Autodesk Inventor part; units mm, degrees
ref_plane "YZ Plane" through (0, 0, 0) normal (1, 0, 0) x (0, 1, 0)
ref_plane "XZ Plane" through (0, 0, 0) normal (0, 1, 0) x (-1, 0, 0)
ref_plane "XY Plane" through (0, 0, 0) normal (0, 0, 1) x (1, 0, 0)
sketch "스케치1" plane through (0, 0, 0) normal (0, 1, 0) x (-1, 0, 0)
  line L0 (-29.3, -54.1) -> (29.3, -54.1)
  line L1 (29.3, -54.1) -> (29.3, 54.1)
  line L2 (29.3, 54.1) -> (-29.3, 54.1)
  line L3 (-29.3, 54.1) -> (-29.3, -54.1)
  line L4 (-29.3, -54.1) -> (29.3, 54.1) construction
  line L5 (29.3, -54.1) -> (-29.3, 54.1) construction
  line L6 (34.5, 59.3) -> (34.5, -59.3)
  line L7 (34.5, -59.3) -> (-34.5, -59.3)
  line L8 (-34.5, -59.3) -> (-34.5, 59.3)
  line L9 (-34.5, 59.3) -> (34.5, 59.3)
  line L10 (34.5, 19.8) -> (29.3, 19.8)
  line L11 (29.3, 19.8) -> (29.3, -19.8)
  line L12 (29.3, -19.8) -> (34.5, -19.8)
  line L13 (34.5, -19.8) -> (34.5, 19.8)
  line L14 (34.5, 19.8) -> (29.3, -19.8) construction
  line L15 (29.3, 19.8) -> (34.5, -19.8) construction
  line L16 (0, 0) -> (0, -10.2235)
  line L17 (31.9, 19.8) -> (31.9, -19.8)
  line L18 (-34.5, 19.8) -> (-29.3, 19.8)
  line L19 (-29.3, 19.8) -> (-29.3, -19.8)
  line L20 (-29.3, -19.8) -> (-34.5, -19.8)
  line L21 (-34.5, -19.8) -> (-34.5, 19.8)
  line L22 (-34.5, 19.8) -> (-29.3, -19.8) construction
  line L23 (-29.3, 19.8) -> (-34.5, -19.8) construction
  line L24 (-31.9, 19.8) -> (-31.9, -19.8)
  point P0 (31.9, 0)
  point P1 (-31.9, 0)
  point P2 (-34.5, 19.8)
  point P3 (-34.5, -19.8)
  dimension "d0" = 58.6
  dimension "d1" = 108.2
  dimension "d4" = 5.2
  dimension "d7" = 39.6
extrude "돌출1" add sketch "스케치1" against normal blind 5
extrude "돌출2" add sketch "스케치1" along normal blind 19.7 contours L20 L8 L18 L24 | L17 L10 L6 L12
chamfer "모따기1" distance 5 angle 45 4 edges at (-34.5, -2.5, 59.3) (34.5, -2.5, 59.3) (34.5, -2.5, -59.3) (-34.5, -2.5, -59.3)
sketch "스케치2" plane through (34.5, 0, -19.8) normal (1, 0, 0) x (0, 0, -1)
  circle A0 centre (-4.8, 15) radius 1
  line L0 (-19.8, 0) -> (-19.8, 7.8444)
  line L1 (-39.6, 19.7) -> (0, 19.7)
  line L2 (-39.6, 0) -> (0, 0)
  circle A1 centre (-34.8, 15) radius 1
  dimension "d14" = 15
  dimension "d15" = 2
  dimension "d16" = 15
extrude "돌출3" cut sketch "스케치2" against normal up to surface (69 mm away)
extrude "돌출4" add sketch "스케치1" along normal blind 3 contours L3 L2 L1 L0
chamfer "모따기2" distance 2 angle 45 4 edges at (-29.3, 1.5, -54.1) (-29.3, 1.5, 54.1) (29.3, 1.5, -54.1) (29.3, 1.5, 54.1)
chamfer "모따기3" distance 2 angle 45 8 edges at (34.5, -5, 0) (32, -5, -56.8) (0, -5, -59.3) (-34.5, -5, 0) (-32, -5, -56.8) (32, -5, 56.8) (0, -5, 59.3) (-32, -5, 56.8)
fillet "모깎기2" radius 1 2 edges at (31.9, 0, 0) (-31.9, 0, 0)
properties part number "컨버터 커버"
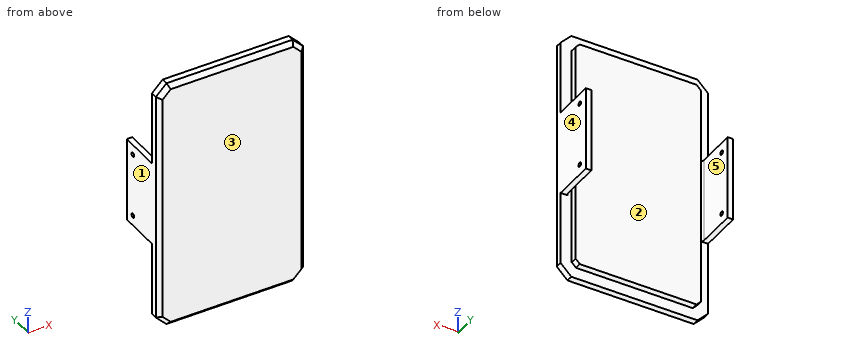
Check sheet for the modelled part. Datum: model origin and axes. Units: mm. Face numbers are marked on the shaded views. A direction names the side the tool comes from. Round coordinates to 2 decimals unless told otherwise and drop trailing zeros. Order: outer loops, then holes, each group sorted by start corner. A loop starts at its lowest first (then second) coordinate and runs counter-clockwise, first axis right, second up.
Q1. Cross-section at C-C, the plane x = -19.5. Enter the section's corners in (y, z), plus the area to 3 significant figures.
Filled sheet:
outline: (-5, -57.3) - (-3, -59.3) - (0, -59.3) - (0, -54.1) - (3, -54.1) - (3, 54.1) - (0, 54.1) - (0, 59.3) - (-3, 59.3) - (-5, 57.3) - close
area: 914 mm2
Q2. Depth check by flat-ended pin: P1, Ø3, axis at x = 32.5, y = 8, coming from the -Z side; P2, Ø1.1, axis at x = 32.5, y = 10.5, coming from the +Z side; P3, Ø20.5, axis at x = -1.5, z = 13, coming from the +Y side; P4, Ø1.8, axis at y = 15, z = 15, coming from the +X side. Enter the tip coordinate at first touch or a pass-through.
Filled sheet:
P1: stops at z = -19.8
P2: stops at z = 19.8
P3: stops at y = 3
P4: passes through
Q3. Cross-section at A-A, the plane y = 10. Enter the section's corners in (x, z).
Filled sheet:
outline: (-34.5, -19.8) - (-31.9, -19.8) - (-31.9, 19.8) - (-34.5, 19.8) - close; (31.9, -19.8) - (34.5, -19.8) - (34.5, 19.8) - (31.9, 19.8) - close
Q4. Set-up check for the marked faces 4 and 5: record each of +Z, -Z, +X, -X, +Y, -Y from which the full face is reachable in a straight line by a thin tool's end or side.
Filled sheet:
face 4: +Z, -Z, +X, +Y, -Y
face 5: +Z, -Z, +Y
Q5. Cross-section at D-D, the plane z = -7.5. Enter the section's corners in (x, y).
Filled sheet:
outline: (-34.5, -3) - (-32.5, -5) - (32.5, -5) - (34.5, -3) - (34.5, 19.7) - (31.9, 19.7) - (31.9, 1) arc R1 cw to (30.9, 0) - (29.3, 0) - (29.3, 3) - (-29.3, 3) - (-29.3, 0) - (-30.9, 0) arc R1 cw to (-31.9, 1) - (-31.9, 19.7) - (-34.5, 19.7) - close
Q6. Scan lines: L1, parallel to X at y = 1.5, z = -16; L2, parallel to X at y = 16.5, z = -16; L3, parallel to Y at x = 12, z = -15. Record each from-to range of solid material in increasing order.
Filled sheet:
L1: x = -34.5 to -31.9, -29.3 to 29.3, 31.9 to 34.5
L2: x = -34.5 to -31.9, 31.9 to 34.5
L3: y = -5 to 3
Q7. Cross-section at B-B, the plane z = 48. Enter the section's corners in (x, y).
Filled sheet:
outline: (-34.5, -3) - (-32.5, -5) - (32.5, -5) - (34.5, -3) - (34.5, 0) - (29.3, 0) - (29.3, 3) - (-29.3, 3) - (-29.3, 0) - (-34.5, 0) - close
Q8. Draft check along X on the marked faces 1, 2 and 3. Enter one of: pulls with the +X half, pulls with the -X half, needs draft (parallel to the pull), parting line crosses it, or undercut.
Filled sheet:
face 1: pulls with the -X half
face 2: undercut
face 3: needs draft
